```python
from build123d import *

# Parameters (mm, degrees)
SKETCH_R     = 3.96875
PAD_DEPTH    = 3.175
SKETCH001_R  = 3.175
PAD001_DEPTH = 6.35
SKETCH002_R  = 3.175
PAD002_DEPTH = 3.175
CHAMFER_SIZE = 2.032


with BuildPart() as part:
    # Sketch → Pad (new body)
    with BuildSketch(Plane.XY):
        Circle(SKETCH_R)
    extrude(amount=PAD_DEPTH)

    # Sketch001 → Pad001 (new body)
    with BuildSketch(Plane.XY.offset(3.175)):
        Circle(SKETCH001_R)
    extrude(amount=PAD001_DEPTH)

    # Sketch002 → Pad002 (new body)
    with BuildSketch(Plane.XY.offset(9.525)):
        Circle(SKETCH002_R)
    extrude(amount=PAD002_DEPTH)

    # Chamfer
    chamfer_edges = [part.edges().sort_by_distance(p)[0] for p in [
        (-3.175, 0, 9.525),
        (-3.175, 0, 12.7),
    ]]
    chamfer(chamfer_edges, length=CHAMFER_SIZE)


solid = part.part
```
Input: part model. Units: mm. Frame: model coordinates. A direction names the side the tool comes from. Give positions to 0.01 mm unless a question says otherwise; leave off trailing zeros. Order: outer loops, then holes, each group sorted by start corner. A loop starts at its lowest first (then second) coordinate and runs counter-clockwise, first axis right, second up. Notation, with made-up numbers: (-29.5, -24) -> (8.5, -24) arc R25 ccw to (8.5, -11) -> close; hole circle Ø9 at (-2.5, 89). An arc over 180 degrees is marked (long way). Write each question's results on one line, items separated by ' | '. Start each with the question number.
Item 1: Cut plane A-A on x = 0. Return the cut outline in (y, z) (3 decimals), then the cut area to 3 significant figures.
Item 2: Contact query for flat-ended pins moving along their axis: P1, Ø2, axis at x = -3, z = 9.5, coming from the +Y side; P2, Ø3, axis at x = 1.5, y = -1, coming from the -Z side; P3, Ø2, axis at x = 0.5, z = 4.5, coming from the +Y side (3 decimals); P4, Ø1.5, axis at x = -2, y = -1.5, coming from the +Z side. Output: stop coordinate, or through.
Item 3: Cut plane B-B on z = 6.75. Return the cut outline in (x, y) (3 decimals).
Item 4: Set-up query: faces 1 (the flat face through (0, 0, 0)), 2 (the flat face through (-2, 3, 3.175)). Return all of +Z, -Z, +X, -X, +Y, -Y with unobstructed straight access to the full face (end or side cutting, diameter ignored); none if empty.
Item 5: Cut plane C-C on z = 1. Return the cut outline in (x, y).
Item 6: Line query: line 1 (Z direction, x = 1.75, y = -3) (3 decimals); line 2 (X direction, y = 3.5, z = 3); line 3 (Y direction, x = 1, z = 4.75). Output: solid intervals per line, ascending.
Established:
1) outline: (-3.969, 0) -> (3.969, 0) -> (3.969, 3.175) -> (3.175, 3.175) -> (3.175, 10.668) -> (1.143, 12.7) -> (-1.143, 12.7) -> (-3.175, 10.668) -> (-3.175, 3.175) -> (-3.969, 3.175) -> close | area: 81.6 mm^2
2) P1: y = 2.47 | P2: z = 0 | P3: y = 3.175 | P4: z = 12.09
3) outline: circle Ø6.35 at (0, 0)
4) face 1: -Z, +X, -X, +Y, -Y | face 2: +Z
5) outline: circle Ø7.94 at (0, 0)
6) line 1: 0 to 3.175 | line 2: -1.87 to 1.87 | line 3: -3.01 to 3.01
